Source: CAD feature listing. Evaluate the final solid. Frame: model axes, mm. Face numbers are marked on the shaded views. A direction names the side the tool comes from. Give positions to 0.01 mm unless a question says otherwise; leave off trailing zeros. Order: outer loops, then holes, each group sorted by start corner. A loop starts at its lowest first (then second) coordinate and runs counter-clockwise, first axis right, second up.
1) Section B-B, the plane y = 0. Return loops of the section in (x, z).
2) Draft query along Z for the marked faces 1, 2 and 3. Return one class per face: released by +Z, released by -Z, zero draft, split by the parting line, or undercut.
3) Access query for the marked faces 4 and 5. Directions: +Z, -Z, +X, -X, +Y, -Y. A direction counts if a zero-diameter tool reaches every point of the face in a straight line with its end or side. Return the directions, or none.
4) Section D-D, the plane y = -88.5. Return loops of the section in (x, z).
5) Material intervals for line 1 (Y direction, x = 26, z = 70); line 2 (Z direction, x = -32, y = -84); line 3 (Y direction, x = -17, z = 65), sorted ascending.
6) First-contact query: P1, Ø14, axis at x = -13.5, y = -84.5, coming from the +Z side; P2, Ø10, axis at x = -3.5, y = -16, coming from the +Z side; P3, Ø10, axis at x = 30.5, z = 55.5, coming from the +Y side. Flat tips, straight axial feed; report the tip coordinate or a pass-through.
7) Section A-A, the plane x = 1. Return loops of the section in (y, z).
8) Section C-C, the plane x = 12.5. Return loops of the section in (y, z).
```python
from build123d import *

# Parameters (mm, degrees)
SKETCH_1_W          = 94.5
SKETCH_1_H          = 255
EXTRUDE_1_DEPTH     = 137
SKETCH_2_OUTSIDE_W  = 199.902
SKETCH_2_OUTSIDE_H  = 317.902
CUT_EXTRUDE_1_DEPTH = 137
FILLET_1_R          = 10
FILLET_2_R          = 5
SKETCH_3_R          = 25
CUT_EXTRUDE_2_DEPTH = 210.655670133
CUT_EXTRUDE_3_DEPTH = 23


with BuildPart() as part:
    # 草图1 → 凸台-拉伸1 (new body)
    with BuildSketch(Plane.XY):
        Rectangle(SKETCH_1_W, SKETCH_1_H)
    extrude(amount=EXTRUDE_1_DEPTH)

    # 草图2 outside → 切除-拉伸1 (cut)
    with BuildSketch(Plane(origin=(47.25, 0, 0), x_dir=(0, 0, -1), z_dir=(1, 0, 0))):
        with Locations((-68.5, 0)):
            Rectangle(SKETCH_2_OUTSIDE_W, SKETCH_2_OUTSIDE_H)
        with BuildLine():
            Line((0, -127.5), (0, 127.5))
            Line((0, 127.5), (-23, 127.5))
            Line((-23, 127.5), (-23, 51.205468458))
            ThreePointArc((-23, 51.205468458), (-137, 0), (-23, -51.205468458))
            Line((-23, -51.205468458), (-23, -127.5))
            Line((-23, -127.5), (0, -127.5))
        make_face(mode=Mode.SUBTRACT)
    extrude(amount=-CUT_EXTRUDE_1_DEPTH, mode=Mode.SUBTRACT)

    # 圆角1
    fillet_1_edges = [part.edges().sort_by_distance(p)[0] for p in [
        (0, 127.5, 23),
        (0, -51.205468458, 23),
        (0, 51.205468458, 23),
        (0, -127.5, 23),
    ]]
    fillet(fillet_1_edges, radius=FILLET_1_R)

    # 圆角2
    fillet_2_edges = [part.edges().sort_by_distance(p)[0] for p in [
        (47.25, 127.5, 6.5),
        (-47.25, 127.5, 6.5),
        (47.25, -93.757142128, 23),
        (47.25, -127.5, 6.5),
        (47.25, 93.757142128, 23),
        (47.25, 0, 137),
        (47.25, -124.571067812, 20.071067812),
        (47.25, 124.571067812, 20.071067812),
        (-47.25, 93.757142128, 23),
        (-47.25, -93.757142128, 23),
        (-47.25, 0, 137),
        (-47.25, -127.5, 6.5),
        (-47.25, -124.571067812, 20.071067812),
        (-47.25, 124.571067812, 20.071067812),
        (47.25, 61.493048139, 27.766594318),
        (-47.25, 61.493048139, 27.766594318),
        (47.25, -61.493048139, 27.766594318),
        (-47.25, -61.493048139, 27.766594318),
    ]]
    fillet(fillet_2_edges, radius=FILLET_2_R)

    # 草图3 → 切除-拉伸2 (cut, through all)
    with BuildSketch(Plane(origin=(47.25, 0, 0), x_dir=(0, 0, -1), z_dir=(1, 0, 0))):
        with Locations((-70, 0)):
            Circle(SKETCH_3_R)
    extrude(amount=-CUT_EXTRUDE_2_DEPTH, mode=Mode.SUBTRACT)

    # 草图4 → 切除-拉伸3 (cut)
    with BuildSketch(Plane(origin=(0, 0, 0), x_dir=(-1, 0, 0), z_dir=(0, 0, -1))):
        with BuildLine():
            Line((9, 107.5), (9, 102.5))
            ThreePointArc((9, 102.5), (0, 93.5), (-9, 102.5))
            Line((-9, 102.5), (-9, 107.5))
            ThreePointArc((-9, 107.5), (0, 116.5), (9, 107.5))
        make_face()
        with BuildLine():
            Line((-9, -107.5), (-9, -102.5))
            ThreePointArc((-9, -102.5), (0, -93.5), (9, -102.5))
            Line((9, -102.5), (9, -107.5))
            ThreePointArc((9, -107.5), (0, -116.5), (-9, -107.5))
        make_face()
    extrude(amount=-CUT_EXTRUDE_3_DEPTH, mode=Mode.SUBTRACT)


solid = part.part
```
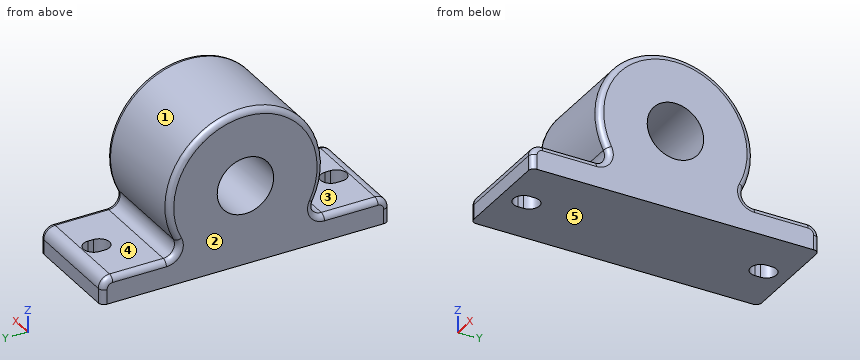
From the geometry:
1. outline: (-47.25, 0) - (47.25, 0) - (47.25, 45) - (-47.25, 45) - close; (-47.25, 95) - (47.25, 95) - (47.25, 132) arc R5 ccw to (42.25, 137) - (-42.25, 137) arc R5 ccw to (-47.25, 132) - close
2. face 1: undercut
2. face 2: zero draft
2. face 3: released by +Z
3. face 4: +Z, +X, -X, +Y
3. face 5: -Z, +X, -X, +Y, -Y
4. outline: (-47.25, 0) - (47.25, 0) - (47.25, 18) arc R5 ccw to (42.25, 23) - (-42.25, 23) arc R5 ccw to (-47.25, 18) - close
5. line 1: y = -68.48 to -25, 25 to 68.48
5. line 2: z = 0 to 23
5. line 3: y = -68.41 to -24.49, 24.49 to 68.41
6. P1: stops at z = 23
6. P2: stops at z = 136.11
6. P3: stops at y = 68.03
7. outline: (-127.5, 0) - (-116.44, 0) - (-116.44, 23) - (-117.5, 23) arc R10 ccw to (-127.5, 13) - close; (-93.56, 0) - (93.56, 0) - (93.56, 23) - (70.01, 23) arc R10 cw to (61.1, 37.52) arc R68.5 ccw (long way) to (-61.1, 37.52) arc R10 cw to (-70.01, 23) - (-93.56, 23) - close; (116.44, 0) - (127.5, 0) - (127.5, 13) arc R10 ccw to (117.5, 23) - (116.44, 23) - close; hole circle Ø50 at (0, 70)
8. outline: (-127.5, 0) - (127.5, 0) - (127.5, 13) arc R10 ccw to (117.5, 23) - (70.01, 23) arc R10 cw to (61.1, 37.52) arc R68.5 ccw (long way) to (-61.1, 37.52) arc R10 cw to (-70.01, 23) - (-117.5, 23) arc R10 ccw to (-127.5, 13) - close; hole circle Ø50 at (0, 70)
